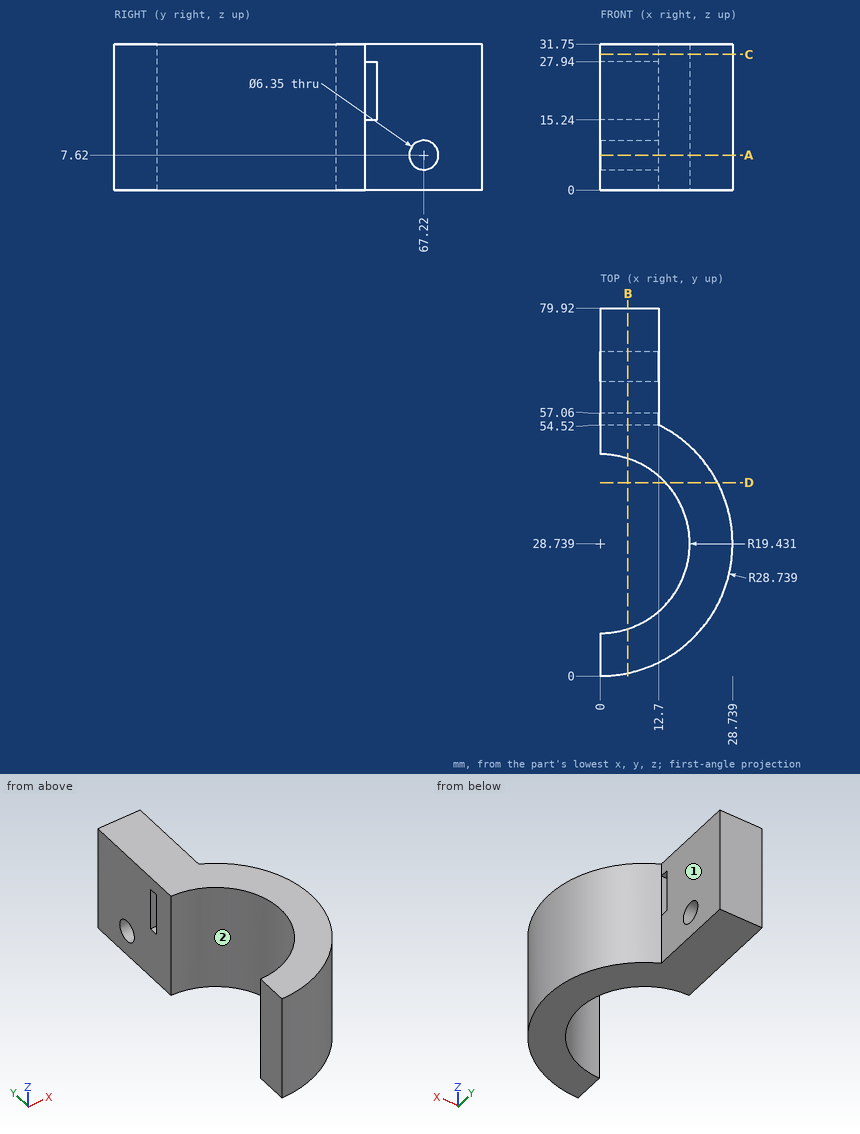
Drawing for the job (mm, zero at the part's lowest x, y, z). A direction names the side the tool comes from. Give positions to 0.01 mm unless a question says otherwise; leave off trailing zeros. Order: outer loops, then holes, each group sorted by start corner. A loop starts at its lowest first (then second) coordinate and runs counter-clockwise, first axis right, second up. Notation, with made-up numbers: M 9.5,53 L 26.5,53 A38 cw 26.5,91 Z; hole C 37,3.25 d10. An arc over 180 degrees is marked long. Use a Markdown table: item, result. Add a question column.
(1) Saw through at A-A, the plane z = 7.62. Give the cut face in (x, y) (1 decimal).
(2) Saw through at C-C, the plane z = 29.5. Give the cut face in (x, y), and give its area (3 significant figures).
(3) Saw through at B-B, the plane x = 6. Give the number of separate pieces and of enclosed holes in the cut face, and give its area (3 significant figures).
(4) Drop flat-ended pins along their axis: P1, Ø5, axis at y = 44, z = 20, coming from the -X side; P2, Ø5, axis at y = 67.22, z = 7.62, coming from the -X side; P3, Ø5, axis at y = 20.5, z = 18.5, coming from the -X side; P4, Ø1.5, axis at x = 16.5, z = 21.5, coming from the +Y side. Give the stop position or say it passes through.
(5) Probe line 1 along X through (y, z) = (74.5, 22); line 2 along Y through (x, z) = (14.5, 7) (1 decimal); line 3 along Y through (x, z) = (9.75, 28.5) (1 decimal). List the from-to ranges inside material, lowest first. Write a range as [from, to].
(6) Saw through at D-D, the plane y = 42. Give the cut face in (x, z), and give its area (3 significant figures).
(7) 3-axis set-ups, long thin cutter, end or side, ignore diameter. For the marked faces 1 and 2: which of +Z, -Z, +X, -X, +Y, -Y reach the whole face in a straight line?
Answer key:
| question | item | result |
|---|---|---|
| 1 | outline | M 0,0 A28.7 ccw 12.7,54.5 L 12.7,64 L 0,64 L 0,48.2 A19.4 cw 0,9.3 Z; M 0,70.4 L 12.7,70.4 L 12.7,79.9 L 0,79.9 Z |
| 2 | outline | M 0,0 A28.74 ccw 12.7,54.52 L 12.7,79.92 L 0,79.92 L 0,48.17 A19.43 cw 0,9.31 Z |
| 2 | area | 1,000 mm^2 |
| 3 | separate pieces | 2 |
| 3 | enclosed holes | 2 |
| 3 | area | 1,280 mm^2 |
| 4 | P1 | x = 7.88 |
| 4 | P2 | through |
| 4 | P3 | x = 16.19 |
| 4 | P4 | y = 52.78 |
| 5 | line 1 | [0, 12.7] |
| 5 | line 2 | [3.9, 15.8], [41.7, 53.6] |
| 5 | line 3 | [1.7, 11.9], [45.5, 79.9] |
| 6 | outline | M 14.2,0 L 25.5,0 L 25.5,31.75 L 14.2,31.75 Z |
| 6 | area | 359 mm^2 |
| 7 | face 1 | +Z, -Z, +X, +Y |
| 7 | face 2 | +Z, -Z, -X |
